Work out the finished part from the listing and answer in its coordinate system (mm). Face numbers are marked on the shaded views. Round coordinates to 2 decimals unless told otherwise and drop trailing zeros. Order: outer loops, then holes, each group sorted by start corner. A loop starts at its lowest first (then second) coordinate and runs counter-clockwise, first axis right, second up. Notation, with made-up numbers: M 10.25,86.25 L 56.25,86.25 A33 ccw 56.25,121.25 Z; hole C 30.5,78 d6. An arc over 180 degrees is marked long. Return JSON: item names as keys, results as strings.
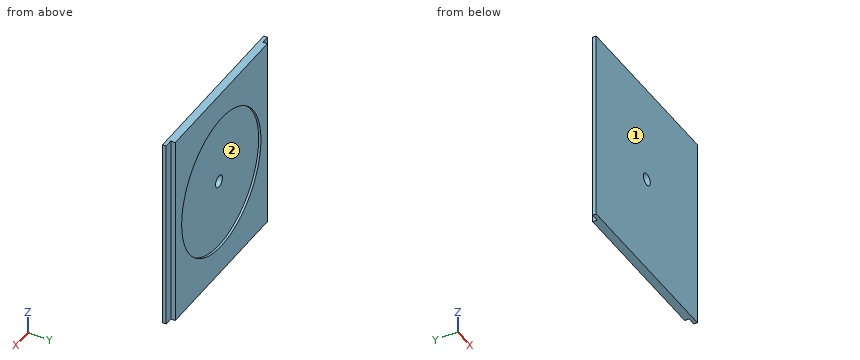
from build123d import *

# Parameters (mm, degrees)
SKETCH1_W           = 139.40028
SKETCH1_H           = 152.4
BOSS_EXTRUDE1_DEPTH = 6.35
SKETCH2_W           = 6.35
SKETCH2_H           = 152.4
CUT_EXTRUDE1_DEPTH  = 3.47472
SKETCH3_R           = 54.58206
CUT_EXTRUDE2_DEPTH  = 1.778
SKETCH4_R           = 4.72186
CUT_EXTRUDE3_DEPTH  = 5.572


with BuildPart() as part:
    # Sketch1 → Boss-Extrude1 (new body)
    with BuildSketch(Plane(origin=(0, 0, 0), x_dir=(1, 0, 0), z_dir=(0, 1, 0))):
        with Locations((69.70014, 76.2)):
            Rectangle(SKETCH1_W, SKETCH1_H)
    extrude(amount=BOSS_EXTRUDE1_DEPTH)

    # Sketch2 → Cut-Extrude1 (cut)
    with BuildSketch(Plane(origin=(0, 6.35, 0), x_dir=(1, 0, 0), z_dir=(0, 1, 0))):
        with Locations((3.175, 76.2)):
            Rectangle(SKETCH2_W, SKETCH2_H)
        with Locations((136.22528, 76.2)):
            Rectangle(SKETCH2_W, SKETCH2_H)
    extrude(amount=-CUT_EXTRUDE1_DEPTH, mode=Mode.SUBTRACT)

    # Sketch3 → Cut-Extrude2 (cut)
    with BuildSketch(Plane(origin=(0, 6.35, 0), x_dir=(1, 0, 0), z_dir=(0, 1, 0))):
        with Locations((69.70014, 76.2)):
            Circle(SKETCH3_R)
    extrude(amount=-CUT_EXTRUDE2_DEPTH, mode=Mode.SUBTRACT)

    # Sketch4 → Cut-Extrude3 (cut, through all)
    with BuildSketch(Plane(origin=(0, 4.572, 0), x_dir=(1, 0, 0), z_dir=(0, 1, 0))):
        with Locations((69.70014, 76.2)):
            Circle(SKETCH4_R)
    extrude(amount=-CUT_EXTRUDE3_DEPTH, mode=Mode.SUBTRACT)


solid = part.part
Item 1: Find section B-B (x = 70). Determine the outline of the cut face in (y, z).
Output:
{"outline": "M 0,-152.4 L 6.35,-152.4 L 6.35,-130.78 L 4.57,-130.78 L 4.57,-80.91 L 0,-80.91 Z; M 0,-71.49 L 4.57,-71.49 L 4.57,-21.62 L 6.35,-21.62 L 6.35,0 L 0,0 Z"}
Item 2: Consider line 1 along X through (y, z) = (1.7, -76.2); line 2 along Y through (x, z) = (70, -68); line 3 along X through (y, z) = (3.25, -82.5). Determine where each line is inside the solid, lowest interval first. Write a range as [from, to].
Output:
{"line 1": "x = [0, 64.98], [74.42, 139.4]", "line 2": "y = [0, 4.57]", "line 3": "x = [6.35, 133.05]"}
Item 3: Find section C-C (x = 107.5). Determine the outline of the cut face in (y, z), plus the area to 3 significant figures.
Output:
{"outline": "M 0,-152.4 L 6.35,-152.4 L 6.35,-115.57 L 4.57,-115.57 L 4.57,-36.83 L 6.35,-36.83 L 6.35,0 L 0,0 Z", "area": "828 mm^2"}
Item 4: Find section A-A (z = -76.2). Determine the outline of the cut face in (x, y).
Output:
{"outline": "M 0,0 L 64.98,0 L 64.98,4.57 L 15.12,4.57 L 15.12,6.35 L 6.35,6.35 L 6.35,2.88 L 0,2.88 Z; M 74.42,0 L 139.4,0 L 139.4,2.88 L 133.05,2.88 L 133.05,6.35 L 124.28,6.35 L 124.28,4.57 L 74.42,4.57 Z"}
Item 5: The mould has two halves that part along Z. Classify the marked faces 1 and 2: pulls with the +Z half, pulls with the -Z half, needs draft (parallel to the pull), parting line crosses it, or undercut.
Output:
{"face 1": "needs draft", "face 2": "undercut"}
Item 6: Each of these flat-tipped pins is pushed along its axis until it touches: pin 1 (1.9 mm diameter, centred on x = 2.5, z = -73, fed in from +Y); pin 2 (1.5 mm diameter, centred on y = 5.5, z = -72.5, fed in from +X); pin 3 (1 mm diameter, centred on y = 4, z = -89.5, fed in from -X). Where does it stop, or does it pass through?
Output:
{"pin 1": "stops at y = 2.88", "pin 2": "stops at x = 133.05", "pin 3": "stops at x = 6.35"}
Item 7: Find section D-D (z = -95.5). Determine the outline of the cut face in (x, y), plus the area to 3 significant figures.
Output:
{"outline": "M 0,0 L 139.4,0 L 139.4,2.88 L 133.05,2.88 L 133.05,6.35 L 120.76,6.35 L 120.76,4.57 L 18.64,4.57 L 18.64,6.35 L 6.35,6.35 L 6.35,2.88 L 0,2.88 Z", "area": "660 mm^2"}
